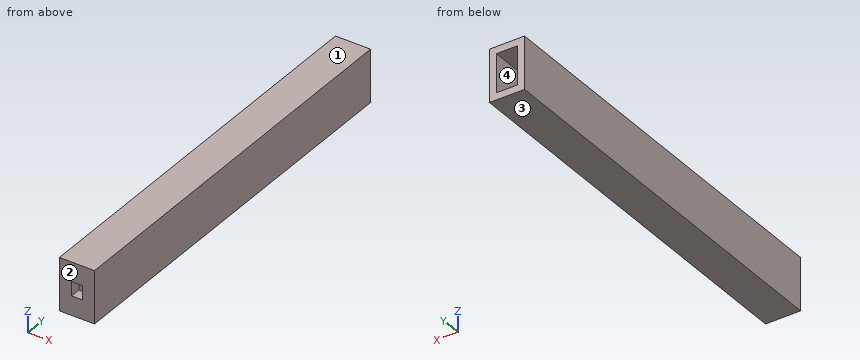
```python
from build123d import *

# Parameters (mm, degrees)
SKETCH1_W           = 10
SKETCH1_H           = 15
BOSS_EXTRUDE1_DEPTH = 115
SKETCH2_W           = 3
SKETCH2_H           = 4
CUT_EXTRUDE1_DEPTH  = 3
SHELL1_START        = 90
SHELL1_OUTLINE_W    = 6
SHELL1_OUTLINE_H    = 11
SHELL1_DEPTH        = 25


# Read off the part's stored shape, not the designer's step: Shell1
with BuildPart() as part:
    # Sketch1 → Boss-Extrude1 (new body)
    with BuildSketch(Plane(origin=(0, 0, 0), x_dir=(1, 0, 0), z_dir=(0, 1, 0))):
        Rectangle(SKETCH1_W, SKETCH1_H)
    extrude(amount=BOSS_EXTRUDE1_DEPTH)

    # Sketch2 → Cut-Extrude1 (cut)
    with BuildSketch(Plane.XZ):
        Rectangle(SKETCH2_W, SKETCH2_H)
    extrude(amount=-CUT_EXTRUDE1_DEPTH, mode=Mode.SUBTRACT)

    # Shell1 outline → Shell1 (cut)
    with BuildSketch(Plane(origin=(0, 0, 0), x_dir=(1, 0, 0), z_dir=(0, 1, 0)).offset(SHELL1_START)):
        Rectangle(SHELL1_OUTLINE_W, SHELL1_OUTLINE_H)
    extrude(amount=SHELL1_DEPTH, mode=Mode.SUBTRACT)


solid = part.part
```
The model under review builds one solid part; all positions refer to its coordinate system, in mm. Face numbers are marked on the shaded views. Coordinates: 2 decimals unless noted, no trailing zeros. Write each loop counter-clockwise with the first axis right and the second up, starting at its lowest first coordinate (ties: lowest second). Pieces come first, ordered by that corner, then holes.
1) To check wall thickness, follow probe 1 along X at (y, z) = (108.5, 1); probe 2 along Z at (x, y) = (-1.25, 105); probe 3 along Y at (x, z) = (-0.75, -3). State the ranges of each line that lie inside material, in increasing order.
2) We need section C-C on z = -1. State the section outline as (x, y) points.
3) We need section A-A on x = 0.5. State the section outline as (y, z) points, then the cut area to 3 significant figures.
4) We need section B-B on y = 102. State the section outline as (x, z) points.
5) Clearance check with flat-ended pins moving along their axes: pin 1 Ø5 at (x, z) = (-2.5, 0) entering from +Y; pin 2 Ø0.9 at (x, z) = (0, 1) entering from -Y; pin 3 Ø3 at (x, z) = (-1, -1) entering from +Y. State where each tip first meets the part, or that it passes through.
6) The part is to be moulded in two halves that separate along Z. For the marked faces 1, 2, 3 and 4, say which applies: pulls with the +Z half, pulls with the -Z half, needs draft (parallel to the pull), parting line crosses it, or undercut.
Answer list:
1. probe 1: x = -5 to -3, 3 to 5
1. probe 2: z = -7.5 to -5.5, 5.5 to 7.5
1. probe 3: y = 0 to 90
2. outline: (-5, 0) - (-1.5, 0) - (-1.5, 3) - (1.5, 3) - (1.5, 0) - (5, 0) - (5, 115) - (3, 115) - (3, 90) - (-3, 90) - (-3, 115) - (-5, 115) - close
3. outline: (0, -7.5) - (115, -7.5) - (115, -5.5) - (90, -5.5) - (90, 5.5) - (115, 5.5) - (115, 7.5) - (0, 7.5) - (0, 2) - (3, 2) - (3, -2) - (0, -2) - close
3. area: 1,440 mm2
4. outline: (-5, -7.5) - (5, -7.5) - (5, 7.5) - (-5, 7.5) - close; hole (-3, -5.5) - (3, -5.5) - (3, 5.5) - (-3, 5.5) - close
5. pin 1: stops at y = 115
5. pin 2: stops at y = 3
5. pin 3: stops at y = 90
6. face 1: pulls with the +Z half
6. face 2: needs draft
6. face 3: pulls with the -Z half
6. face 4: undercut
